Job drawing, mm, ordinate dimensions from the low corner. One solid piece. Round coordinates to 2 decimals unless told otherwise and drop trailing zeros. Order: outer loops, then holes, each group sorted by start corner. A loop starts at its lowest first (then second) coordinate and runs counter-clockwise, first axis right, second up. Notation, with made-up numbers: (-17.5, 78) -> (5.5, 78) arc R8 ccw to (5.5, 84) -> close; hole circle Ø5 at (-17.5, 41). An arc over 180 degrees is marked (long way). Write item = value, one per line.
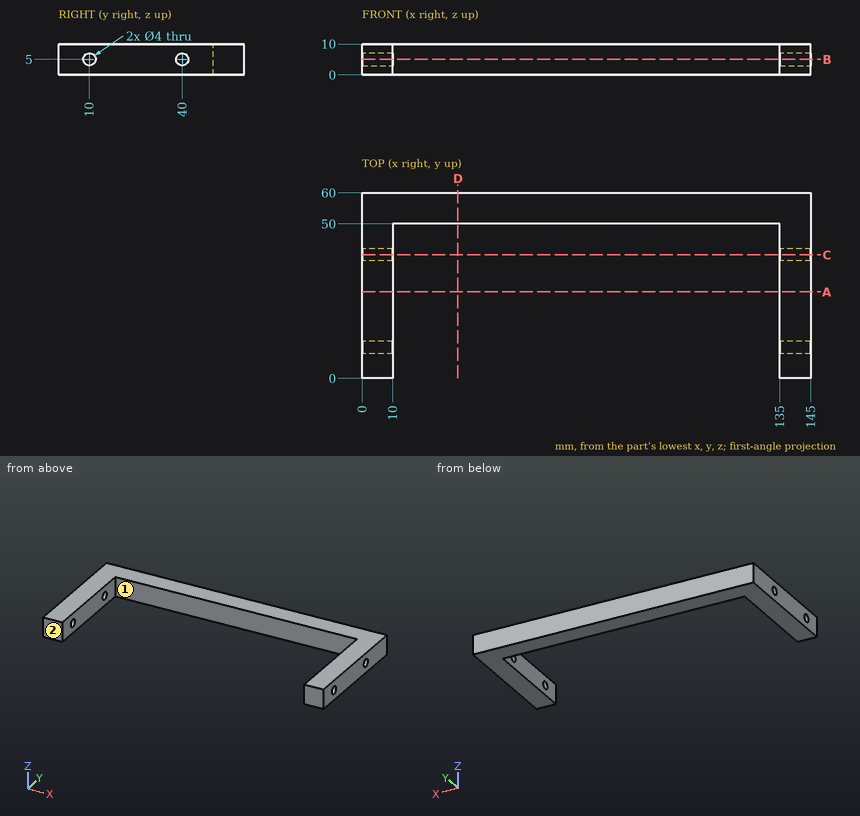
Q1. Cut at D-D, the plane x = 31. List the corners of the cut face in (y, z).
Check values:
outline = (50, 0) -> (60, 0) -> (60, 10) -> (50, 10) -> close
Q2. Flat gauge pins, fed straight in: pin 1 (2.5 mm diameter, centred on y = 40, z = 5, fed in from +X); pin 2 (3 mm diameter, centred on x = 63, z = 6, fed in from -Y). Where does each tip first touch, or does it go through?
Check values:
pin_1 = through
pin_2 = 50
Q3. Cut at C-C, the plane y = 40. List the corners of the cut face in (x, z), and give its area (3 significant figures).
Check values:
outline = (0, 0) -> (10, 0) -> (10, 3) -> (0, 3) -> close; (0, 7) -> (10, 7) -> (10, 10) -> (0, 10) -> close; (135, 0) -> (145, 0) -> (145, 3) -> (135, 3) -> close; (135, 7) -> (145, 7) -> (145, 10) -> (135, 10) -> close
area = 120 mm²
Q4. Cut at B-B, the plane z = 5. List the corners of the cut face in (x, y).
Check values:
outline = (0, 0) -> (10, 0) -> (10, 8) -> (0, 8) -> close; (0, 12) -> (10, 12) -> (10, 38) -> (0, 38) -> close; (0, 42) -> (10, 42) -> (10, 50) -> (135, 50) -> (135, 42) -> (145, 42) -> (145, 60) -> (0, 60) -> close; (135, 0) -> (145, 0) -> (145, 8) -> (135, 8) -> close; (135, 12) -> (145, 12) -> (145, 38) -> (135, 38) -> close
Q5. Mould opens along X. For the marked faces 1 and 2 say: released by +X, released by -X, zero draft, split by the parting line, or undercut.
Check values:
face_1 = undercut
face_2 = zero draft
Q6. Cut at A-A, the plane y = 28. List the corners of the cut face in (x, z).
Check values:
outline = (0, 0) -> (10, 0) -> (10, 10) -> (0, 10) -> close; (135, 0) -> (145, 0) -> (145, 10) -> (135, 10) -> close
Q7. Probe probe 1 along Y at (x, z) = (138.5, 5); probe 2 along X at (y, z) = (30.5, 1.25); probe 3 along Z at (x, y) = (5.5, 40). List the from-to ranges inside material, lowest first.
Check values:
probe_1 = 0 to 8, 12 to 38, 42 to 60
probe_2 = 0 to 10, 135 to 145
probe_3 = 0 to 3, 7 to 10
